The model under review builds one solid part; all positions refer to its coordinate system, in mm. A direction names the side the tool comes from. Round coordinates to 2 decimals unless told otherwise and drop trailing zeros. Loops run counter-clockwise (first coordinate to the right, second up) from the corner with the lowest first, then second, coordinate; pieces in that order, holes last. Notation, with made-up numbers: M 76.25,60.5 L 91.25,60.5 A24 cw 91.25,75.5 Z; hole C 12.5,-7.75 d4. An arc over 180 degrees is marked long. Answer in a Markdown table with one row per item. Add a question column.
from build123d import *

# Parameters (mm, degrees)
F1_R     = 16.7005
F1_R_2   = 12.065
F3_DEPTH = 6.35
F4_DEPTH = 6.35


with BuildPart() as f2:
    # F2: sweep along a path in F0
    with BuildLine(Plane.YZ) as f2_path:
        ThreePointArc((38.1, 0), (26.9407683632, 26.9407683632), (0, 38.1))
    # F1 (on Front) → F2 (sweep)
    with BuildSketch(Plane.XZ):
        with Locations((0, 38.1)):
            Circle(F1_R)
        with Locations((0, 38.1)):
            Circle(F1_R_2, mode=Mode.SUBTRACT)
    sweep(path=f2_path.line)

    # F3 (add): a face of the model
    f3_faces = [f2.faces().sort_by_distance(p)[0] for p in [
        (-16.228138528, 0, 38.1),
    ]]
    extrude(f3_faces, amount=F3_DEPTH)

    # F4 (add): a face of the model
    f4_faces = [f2.faces().sort_by_distance(p)[0] for p in [
        (-16.228138528, 38.1, 0),
    ]]
    extrude(f4_faces, amount=F4_DEPTH)


solid = f2.part
1. To check wall thickness, follow probe 1 along X at (y, z) = (38.1, -4) (1 decimal); probe 2 along Y at (x, z) = (0, -1) (1 decimal). State the ranges of each line that lie inside material, in increasing order.
2. For pin 1 Ø6 at (x, y) = (4, 7.5) entering from -Z; pin 2 Ø6 at (x, y) = (-8.5, 12) entering from -Z; pin 3 Ø10 at (y, z) = (40, 0) entering from +X; pin 4 Ø12 at (x, y) = (10, 35) entering from +Z, all flat-tipped, find the tip position at first contact; note any pin that passes through.
3. Take a section at B-B, the plane z = -1. State the section outline as (x, y) points (1 decimal).
4. Machinability: for faces 5 (the flat face through (-9, 47, -6.35)), 6 (the cylindrical face through (15.93, -3.13, 33.08)), which of the approach directions +Z, -Z, +X, -X, +Y, -Y give a long, thin tool a straight path to every point of the face, cutting with its end or side? Answer none if there is none.
5. Mouldability with a two-part tool opening along X and no side actions: class faces 1 (the cylindrical face through (6.49, 27.93, -3.13)), 2 (the flat face through (8.7, -6.35, 29.5)), 3 (the cylindrical face through (-3.62, 54.403, -3.131)), 4 (the cylindrical face through (6.49, -3.13, 27.93)) as released by +X, released by -X, zero draft, split by the parting line, or undercut.
6. Take a section at C-C, the plane x = 9.5. State the section outline as (y, z) points.
Check sheet entries:
| question | item | result |
|---|---|---|
| 1 | probe 1 | x = -16.7 to -12.1, 12.1 to 16.7 |
| 1 | probe 2 | y = 21.4 to 26, 50.2 to 54.8 |
| 2 | pin 1 | stops at z = 19.05 |
| 2 | pin 2 | stops at z = 17.68 |
| 2 | pin 3 | stops at x = 16.7 |
| 2 | pin 4 | stops at z = 44.19 |
| 3 | outline | C 0,38.1 d33.4; hole C 0,38.1 d24.1 |
| 4 | face 5 | -Z, +X, -X, +Y, -Y |
| 4 | face 6 | -Y |
| 5 | face 1 | undercut |
| 5 | face 2 | zero draft |
| 5 | face 3 | split by the parting line |
| 5 | face 4 | undercut |
| 6 | outline | M -6.35,24.36 L 0,24.36 A24.36 cw 24.36,0 L 24.36,-6.35 L 30.66,-6.35 L 30.66,0 A30.66 ccw 0,30.66 L -6.35,30.66 Z; M -6.35,45.54 L 0,45.54 A45.54 cw 45.54,0 L 45.54,-6.35 L 51.84,-6.35 L 51.84,0 A51.84 ccw 0,51.84 L -6.35,51.84 Z |
